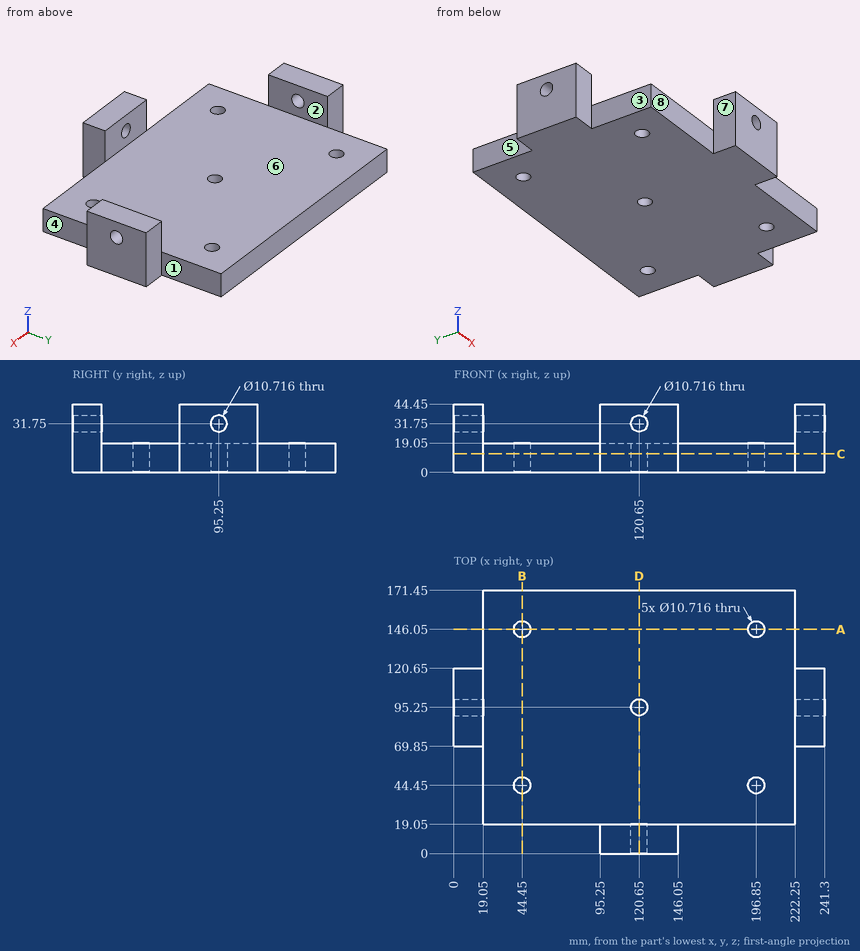
Can you work these out from the drawing? Everything is in mm from the part's minimum corner. A direction names the side the tool comes from. Round coordinates to 2 decimals unless told otherwise and drop trailing zeros. Write each loop counter-clockwise with the first axis right and the second up, starting at its lowest first coordinate (ties: lowest second). Pieces come first, ordered by that corner, then holes. Notation, with made-up numbers: (16.25, -21) - (21.25, -21) arc R15 ccw to (21.25, -9) - close; hole circle Ø10 at (5, 17). An arc over 180 degrees is marked (long way). Write each question's results on one line, items separated by ' | '. Start each with the question number.
1) Suppose I cut it at A-A (y = 146.05). List the corners of the cut face in (x, z) for me, and give its area (3 significant figures).
2) Suppose I cut it at C-C (z = 12). List the corners of the cut face in (x, y) for me.
3) Which directions (+Z, -Z, +X, -X, +Y, -Y) give clear straight access to the entire face, cutting with the end or side of a thin tool? Please do the marked faces 1, 2, 3, 4 and 5.
4) Please list where these lines run through material, in increasing order: line 1 (X direction, y = 44, z = 6); line 2 (X direction, y = 96.5, z = 22); line 3 (Z direction, x = 120.65, y = 7.75).
5) Suppose I cut it at D-D (x = 120.65). List the corners of the cut face in (y, z) for me.
6) Suppose I cut it at B-B (x = 44.45). List the corners of the cut face in (y, z) for me.
7) For pin 1 Ø1 at (x, z) = (99, 39) entering from -Y; pin 2 Ø12.5 at (x, y) = (44.45, 146.05) entering from +Z; pin 3 Ø9.5 at (y, z) = (146.5, 10.5) entering from +X; pin 4 Ø21 at (x, z) = (12.5, 19) entering from -Y, each with a flat end and sliding along its axis, tell me the tip position at first contact or that it passes through.
8) We'd pull the mould along X, two halves only. Please class the marked faces 6, 7 and 8: released by +X, released by -X, zero draft, split by the parting line, or undercut.
Here are the results:
1) outline: (19.05, 0) - (39.09, 0) - (39.09, 19.05) - (19.05, 19.05) - close; (49.81, 0) - (191.49, 0) - (191.49, 19.05) - (49.81, 19.05) - close; (202.21, 0) - (222.25, 0) - (222.25, 19.05) - (202.21, 19.05) - close | area: 3,460 mm2
2) outline: (0, 69.85) - (19.05, 69.85) - (19.05, 19.05) - (95.25, 19.05) - (95.25, 0) - (146.05, 0) - (146.05, 19.05) - (222.25, 19.05) - (222.25, 69.85) - (241.3, 69.85) - (241.3, 120.65) - (222.25, 120.65) - (222.25, 171.45) - (19.05, 171.45) - (19.05, 120.65) - (0, 120.65) - close; hole circle Ø10.72 at (44.45, 44.45); hole circle Ø10.72 at (44.45, 146.05); hole circle Ø10.72 at (120.65, 95.25); hole circle Ø10.72 at (196.85, 44.45); hole circle Ø10.72 at (196.85, 146.05)
3) face 1: +Z, -Z, +X, +Y | face 2: +Z, +Y, -Y | face 3: +Z, -Z, -X, -Y | face 4: +Z, -Z, +X, -Y | face 5: +Z, -Z, -X, +Y
4) line 1: x = 19.05 to 39.11, 49.79 to 191.51, 202.19 to 222.25 | line 2: x = 0 to 19.05, 222.25 to 241.3 | line 3: z = 0 to 26.39, 37.11 to 44.45
5) outline: (0, 0) - (89.89, 0) - (89.89, 19.05) - (19.05, 19.05) - (19.05, 26.39) - (0, 26.39) - close; (0, 37.11) - (19.05, 37.11) - (19.05, 44.45) - (0, 44.45) - close; (100.61, 0) - (171.45, 0) - (171.45, 19.05) - (100.61, 19.05) - close
6) outline: (19.05, 0) - (39.09, 0) - (39.09, 19.05) - (19.05, 19.05) - close; (49.81, 0) - (140.69, 0) - (140.69, 19.05) - (49.81, 19.05) - close; (151.41, 0) - (171.45, 0) - (171.45, 19.05) - (151.41, 19.05) - close
7) pin 1: stops at y = 0 | pin 2: stops at z = 19.05 | pin 3: stops at x = 222.25 | pin 4: stops at y = 19.05
8) face 6: undercut | face 7: released by -X | face 8: zero draft
